Can you work these out from the model? Positions are in its coordinate system, mm. A direction names the side the tool comes from. Coordinates: 2 decimals unless noted, no trailing zeros. Order: outer loops, then holes, each group sorted by start corner. A loop starts at its lowest first (then second) coordinate and runs counter-clockwise, first axis right, second up. Notation, with made-up numbers: (-15, 41) -> (1, 41) arc R34 ccw to (1, 74) -> close; hole circle Ø1 at (75, 60.5). An arc over 180 degrees is marked (long way). Answer as CSV lines item,"result".
from build123d import *


with BuildPart() as part:
    # Çizim1 → Döndür1 (revolve)
    with BuildSketch(Plane.XY, mode=Mode.PRIVATE) as d_nd_r1_sk:
        Polygon((0, 0), (0, 3.975), (24, 3.975), (24, 6), (28, 6), (28, 16.25), (65.5, 16.25), (65.5, 9), (69.5, 9), (69.5, 7.5), (78, 7.5), (78, 6.975), (108, 6.975), (108, 0), align=None)
    revolve(d_nd_r1_sk.sketch.rotate(Axis((0, 0, 0), (1, 0, 0)), 90), axis=Axis((0, 0, 0), (1, 0, 0)))


solid = part.part
Q1. Which directions (+Z, -Z, +X, -X, +Y, -Y) give clear straight access to the entire face, cutting with the end or side of a thin tool? Please do faces 4 (the cylindrical face through (93.21, 6.81, -1.51)), 5 (the cylindrical face through (12.17, -0.17, -3.97)), 6 (the flat face through (108, 0, 0)).
Solution:
face 4,"+X"
face 5,"-X"
face 6,"+Z, -Z, +X, +Y, -Y"
Q2. Imagine slicing it at A-A (y = 0). List the corners of the cut face in (x, z) for me (3 decimals).
Solution:
outline,"(0, -3.975) -> (24, -3.975) -> (24, -6) -> (28, -6) -> (28, -16.25) -> (65.5, -16.25) -> (65.5, -9) -> (69.5, -9) -> (69.5, -7.5) -> (78, -7.5) -> (78, -6.975) -> (108, -6.975) -> (108, 6.975) -> (78, 6.975) -> (78, 7.5) -> (69.5, 7.5) -> (69.5, 9) -> (65.5, 9) -> (65.5, 16.25) -> (28, 16.25) -> (28, 6) -> (24, 6) -> (24, 3.975) -> (0, 3.975) -> close"
Q3. For P1, Ø6, axis at x = 27, z = -12, coming from the -Y side; P2, Ø5, axis at y = -8, z = 2, coming from the -X side; P3, Ø5, axis at x = 61.5, z = 8.5, coming from the +Y side; P4, Ø6, axis at x = 91.5, y = 12.5, coming from the +Z side, each with a flat end and sliding along its axis, tell me the tip position at first contact or that it passes through.
Solution:
P1,"y = -13.41"
P2,"x = 24"
P3,"y = 15.1"
P4,"through"
Q4. Imagine slicing it at C-C (x = 71). List the corners of the cut face in (y, z) for me.
Solution:
outline,"circle Ø15 at (0, 0)"
Q5. Imagine slicing it at D-D (x = 8). List the corners of the cut face in (y, z) for me (3 decimals), and give its area (3 significant figures).
Solution:
outline,"circle Ø7.95 at (0, 0)"
area,"49.6 mm2"
Q6. We'd pull the mould along X, two halves only. Please class faces 1 (the flat face through (78, 7, 2)), 2 (the flat face through (24, 3.9, 1.4)), 3 (the cylindrical face through (26.028, -1.802, 5.723)): pulls with the +X half, pulls with the -X half, needs draft (parallel to the pull), parting line crosses it, or undercut.
Solution:
face 1,"pulls with the +X half"
face 2,"pulls with the -X half"
face 3,"needs draft"
Q7. If I drill on line 1 (X direction, y = 8.5, z = -5); line 2 (X direction, y = 6.5, z = -3.5); line 3 (Z direction, x = 68, y = -6), over which ranges is the centre line in solid material (lowest first)?
Solution:
line 1,"28 to 65.5"
line 2,"28 to 78"
line 3,"-6.71 to 6.71"
